Verification items for the finished model (mm, model axes). Face numbers are marked on the shaded views. A direction names the side the tool comes from. Coordinates: 2 decimals unless noted, no trailing zeros. Write each loop counter-clockwise with the first axis right and the second up, starting at its lowest first coordinate (ties: lowest second). Pieces come first, ordered by that corner, then holes. Notation, with made-up numbers: (85, 88.5) -> (96, 88.5) arc R18 ccw to (96, 98.5) -> close; hole circle Ø3 at (-20.75, -36). An arc over 180 degrees is marked (long way). Write item = value, one per line. Start each with the question number.
(1) Section check C-C (y = 223). Record the cut outline in (x, z), plus the area to 3 significant figures.
(2) Mould release check, pull along X, two halves, no side actions. Record for the marked faces 6, 7 and 8: released by +X, released by -X, zero draft, split by the parting line, or undercut.
(3) Material ranges on probe 1 along Z at (x, y) = (247, 231); probe 2 along Y at (x, z) = (261.5, 2); probe 3 along X at (y, z) = (227.25, 10.75), recorded low to high. Write a range as [from, to].
(4) Section check B-B (x = 265.5). Record the cut outline in (y, z), plus the area to 3 significant figures.
(5) Section check D-D (z = 7.75). Record the cut outline in (x, y), plus the area to 3 significant figures.
(6) Section check A-A (x = 254.5). Record the cut outline in (y, z), plus the area to 4 significant figures.
(7) Gauge pin test, flat ends, axial feed: pin 1 Ø2 at (x, y) = (242.5, 220) entering from -Z; pin 2 Ø1.6 at (x, z) = (255, 10.5) entering from -Y; pin 3 Ø0.6 at (x, z) = (255, 11.5) entering from +Y; pin 4 Ø2 at (y, z) = (231, 5) entering from -X. Record the tip position at first contact, or that the pin passes through.
(8) Set-up check for the marked faces 1, 2, 3, 4 and 5: record each of +Z, -Z, +X, -X, +Y, -Y from which the full face is reachable in a straight line by a thin tool's end or side.
```python
from build123d import *

# Parameters (mm, degrees)
SKETCH1_W           = 36.5
SKETCH1_H           = 18.5
SKETCH1_R           = 3.45
BOSS_EXTRUDE1_DEPTH = 12.5
SKETCH2_W           = 29.5
SKETCH2_H           = 7
CUT_EXTRUDE1_DEPTH  = 19.5
SKETCH3_R           = 3.45
SKETCH3_R_2         = 2.5
BOSS_EXTRUDE3_DEPTH = 2.75
SKETCH4_W           = 36.5
SKETCH4_H           = 2.75
BOSS_EXTRUDE4_DEPTH = 3
SKETCH5_W           = 36.5
SKETCH5_H           = 2.75
BOSS_EXTRUDE5_DEPTH = 3
CHAMFER1_SIZE       = 3.5
CHAMFER3_SIZE       = 3.5
CUT_EXTRUDE2_DEPTH  = 3
SKETCH7_R           = 2.5
CUT_EXTRUDE3_DEPTH  = 5
FILLET1_R           = 2


with BuildPart() as part:
    # Sketch1 → Boss-Extrude1 (new body)
    with BuildSketch(Plane.XY):
        with Locations((252.305597075, 227.81595418)):
            Rectangle(SKETCH1_W, SKETCH1_H)
        with Locations((239.915979082, 227.815953297)):
            Circle(SKETCH1_R, mode=Mode.SUBTRACT)
        with BuildLine():
            Line((253.99332378, 221.31595418), (255.99332378, 221.31595418))
            ThreePointArc((255.99332378, 221.31595418), (262.49332378, 227.81595418), (255.99332378, 234.31595418))
            Line((255.99332378, 234.31595418), (253.99332378, 234.31595418))
            ThreePointArc((253.99332378, 234.31595418), (247.49332378, 227.81595418), (253.99332378, 221.31595418))
        make_face(mode=Mode.SUBTRACT)
    extrude(amount=BOSS_EXTRUDE1_DEPTH)

    # Sketch2 → Cut-Extrude1 (cut, through all)
    with BuildSketch(Plane(origin=(0, 237.06595418, 0), x_dir=(1, 0, 0), z_dir=(0, 1, 0))):
        with Locations((248.805597075, -6.25)):
            Rectangle(SKETCH2_W, SKETCH2_H)
    extrude(amount=-CUT_EXTRUDE1_DEPTH, mode=Mode.SUBTRACT)

    # Sketch3 → Boss-Extrude3 (add)
    with BuildSketch(Plane.XY.offset(12.5)):
        with Locations((239.915979082, 227.815953297)):
            Circle(SKETCH3_R)
        with Locations((239.915979082, 227.815953297)):
            Circle(SKETCH3_R_2, mode=Mode.SUBTRACT)
    extrude(amount=-BOSS_EXTRUDE3_DEPTH)

    # Sketch4 → Boss-Extrude4 (add)
    with BuildSketch(Plane(origin=(0, 237.06595418, 0), x_dir=(1, 0, 0), z_dir=(0, 1, 0))):
        with Locations((252.305597075, -1.375)):
            Rectangle(SKETCH4_W, SKETCH4_H)
    extrude(amount=BOSS_EXTRUDE4_DEPTH)

    # Sketch5 → Boss-Extrude5 (add)
    with BuildSketch(Plane.XZ.offset(-218.56595418)):
        with Locations((252.305597075, 1.375)):
            Rectangle(SKETCH5_W, SKETCH5_H)
    extrude(amount=BOSS_EXTRUDE5_DEPTH)

    # Chamfer1
    chamfer1_edges = [part.edges().sort_by_distance(p)[0] for p in [
        (270.555597075, 215.56595418, 1.375),
    ]]
    chamfer(chamfer1_edges, length=CHAMFER1_SIZE)

    # Chamfer3
    chamfer3_edges = [part.edges().sort_by_distance(p)[0] for p in [
        (270.555597075, 240.06595418, 1.375),
    ]]
    chamfer(chamfer3_edges, length=CHAMFER3_SIZE)

    # Sketch6 → Cut-Extrude2 (cut)
    with BuildSketch(Plane.ZY.offset(-263.555597075)):
        Polygon((6.25, 224.005442403), (9.55, 225.910698292), (9.55, 229.721210068), (6.25, 231.626465957), (2.95, 229.721210068), (2.95, 225.910698292), align=None)
    extrude(amount=-CUT_EXTRUDE2_DEPTH, mode=Mode.SUBTRACT)

    # Sketch7 → Cut-Extrude3 (cut, through all)
    with BuildSketch(Plane.ZY.offset(-266.555597075)):
        with Locations((6.25, 227.81595418)):
            Circle(SKETCH7_R)
    extrude(amount=-CUT_EXTRUDE3_DEPTH, mode=Mode.SUBTRACT)

    # Fillet1
    fillet1_edges = [part.edges().sort_by_distance(p)[0] for p in [
        (234.055597075, 240.06595418, 1.375),
        (234.055597075, 218.56595418, 11.125),
        (234.055597075, 237.06595418, 11.125),
        (234.055597075, 215.56595418, 1.375),
    ]]
    fillet(fillet1_edges, radius=FILLET1_R)


solid = part.part
```
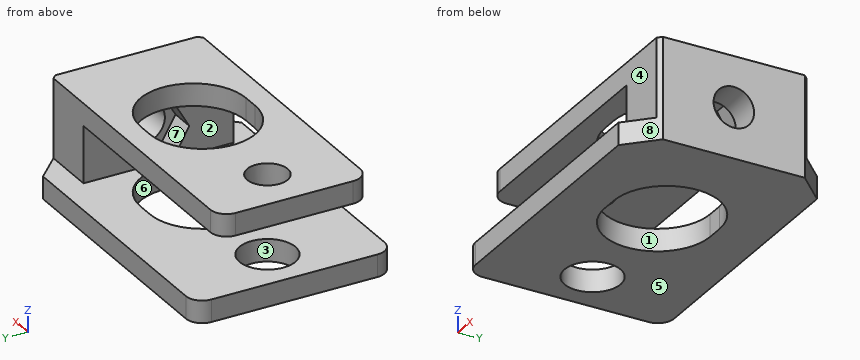
Response:
q1.outline = (234.06, 0) -> (249.63, 0) -> (249.63, 2.75) -> (234.06, 2.75) -> close; (234.06, 9.75) -> (249.63, 9.75) -> (249.63, 12.5) -> (234.06, 12.5) -> close; (260.36, 0) -> (270.56, 0) -> (270.56, 12.5) -> (260.36, 12.5) -> (260.36, 9.75) -> (263.56, 9.75) -> (263.56, 2.75) -> (260.36, 2.75) -> close
q1.area = 191 mm2
q2.face_6 = undercut
q2.face_7 = zero draft
q2.face_8 = released by +X
q3.probe_1 = [0, 2.75], [9.75, 12.5]
q3.probe_2 = [215.57, 224.36], [231.27, 240.07]
q3.probe_3 = [234.06, 237.48], [242.35, 247.52], [262.47, 270.56]
q4.outline = (215.57, 0) -> (240.07, 0) -> (240.07, 2.75) -> (237.07, 2.75) -> (237.07, 12.5) -> (218.57, 12.5) -> (218.57, 2.75) -> (215.57, 2.75) -> close; hole (224.01, 6.25) -> (225.91, 2.95) -> (229.72, 2.95) -> (231.63, 6.25) -> (229.72, 9.55) -> (225.91, 9.55) -> close
q4.area = 210 mm2
q5.outline = (263.56, 218.57) -> (270.06, 218.57) -> (270.56, 219.07) -> (270.56, 225.82) -> (266.56, 225.82) -> (266.56, 224.87) -> (263.56, 224.87) -> close; (263.56, 230.76) -> (266.56, 230.76) -> (266.56, 229.82) -> (270.56, 229.82) -> (270.56, 236.57) -> (270.06, 237.07) -> (263.56, 237.07) -> close
q5.area = 95.6 mm2
q6.outline = (215.57, 0) -> (221.32, 0) -> (221.32, 2.75) -> (215.57, 2.75) -> close; (218.57, 9.75) -> (221.32, 9.75) -> (221.32, 12.5) -> (218.57, 12.5) -> close; (234.32, 0) -> (240.07, 0) -> (240.07, 2.75) -> (234.32, 2.75) -> close; (234.32, 9.75) -> (237.07, 9.75) -> (237.07, 12.5) -> (234.32, 12.5) -> close
q6.area = 46.75 mm2
q7.pin_1 = 0
q7.pin_2 = 218.57
q7.pin_3 = 237.07
q7.pin_4 = 263.56
q8.face_1 = +Z, -Z
q8.face_2 = -X, +Y, -Y
q8.face_3 = -Z
q8.face_4 = +Z, +X, -X, -Y
q8.face_5 = -Z, +X, -X, +Y, -Y
